Could you check a few things on this model? Use its own coordinates, in mm. Face numbers are marked on the shaded views. A direction names the side the tool comes from. Round coordinates to 2 decimals unless told otherwise and drop trailing zeros. Loops run counter-clockwise (first coordinate to the right, second up) from the corner with the lowest first, then second, coordinate; pieces in that order, holes last. Notation, with made-up numbers: (36, -14.5) -> (48, -14.5) arc R27 cw to (48, 9.5) -> close; hole circle Ø6 at (69, -24). An arc over 180 degrees is marked (long way). Write each question's results on one line, items separated by ' | '.
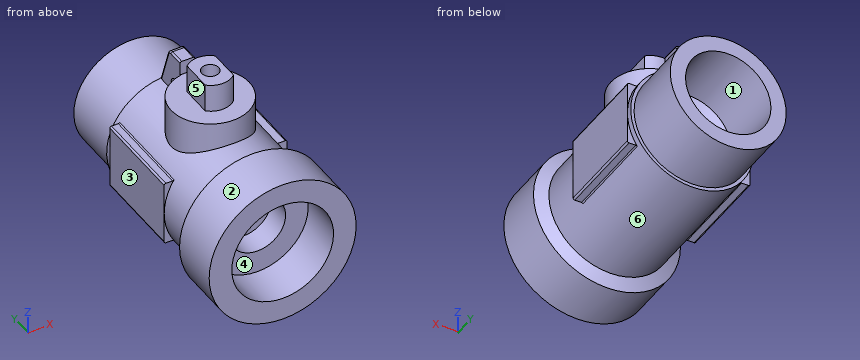
from build123d import *

# Parameters (mm, degrees)
SKETCH2_W                = 16.5
SKETCH2_H                = 11.5
BOSS_EXTRUDE1_DEPTH      = 2
BOSS_EXTRUDE2_DEPTH      = 4.5
BOSS_EXTRUDE2_DEPTH_BACK = 3
SKETCH3_R                = 6.925
BOSS_EXTRUDE6_DEPTH      = 1.3
BOSS_EXTRUDE6_DEPTH_BACK = 1.3
SKETCH4_R                = 1
FILLET2_R                = 0.3
FILLET4_R                = 0.3
FILLET7_R                = 0.3
FILLET8_R                = 0.3
FILLET9_R                = 0.3
FILLET10_R               = 0.3
FILLET11_R               = 0.3
FILLET12_R               = 0.3
SKETCH5_R                = 1.5
BOSS_EXTRUDE7_DEPTH      = 5
FILLET13_R               = 1


with BuildPart() as part:
    # Sketch1 → Revolve1 (revolve)
    with BuildSketch(Plane.XY, mode=Mode.PRIVATE) as revolve1_sk:
        Polygon((7.55, 45.85), (7.55, 33.85), (5, 32.85), (5, 28.85), (0, 28.85), (0, 12), (5, 12), (5, 7.7), (9, 7.7), (9, 0), (13, 0), (13, 9), (10.85, 10), (10.85, 34.85), (10.25, 34.85), (10.25, 45.85), align=None)
    revolve(revolve1_sk.sketch.rotate(Axis((0, 0, 0), (0, 1, 0)), 90), axis=Axis((0, 0, 0), (0, 1, 0)))

    # Sketch2 → Boss-Extrude1 (add)
    with BuildSketch(Plane.YZ.offset(10.85)):
        with Locations((25.6, 0)):
            Rectangle(SKETCH2_W, SKETCH2_H)
    boss_extrude1 = extrude(amount=-BOSS_EXTRUDE1_DEPTH)

    # Mirror1: Boss-Extrude1 across plane
    add(boss_extrude1.mirror(Plane(origin=(0, 0, 0), x_dir=(0, 0, 1), z_dir=(1, 0, 0))))

    # Sketch3 → Boss-Extrude2 (add, two sides: drawn at the far end of the back side and taken through both)
    with BuildSketch(Plane(origin=(0, 0, 10.85), x_dir=(0, -1, 0), z_dir=(0, 0, 1)).offset(-BOSS_EXTRUDE2_DEPTH_BACK)):
        with Locations(Location((-22, 0, 0), (0, 0, 90))):
            Circle(SKETCH3_R)
    extrude(amount=BOSS_EXTRUDE2_DEPTH + BOSS_EXTRUDE2_DEPTH_BACK)

    # Sketch4 → Boss-Extrude6 (add, two sides: drawn at the far end of the back side and taken through both)
    with BuildSketch(Plane(origin=(0, 0, 0), x_dir=(0, 0, -1), z_dir=(1, 0, 0)).offset(-BOSS_EXTRUDE6_DEPTH_BACK)):
        Polygon((-10.85, 34.85), (-17.85, 32.425), (-17.85, 28.925), (-15.35, 28.925), (-15.35, 27.925), (-10.25, 27.925), (-10.25, 34.85), align=None)
        with Locations((-12.35, 30.625)):
            Circle(SKETCH4_R, mode=Mode.SUBTRACT)
    extrude(amount=BOSS_EXTRUDE6_DEPTH + BOSS_EXTRUDE6_DEPTH_BACK)

    # Fillet2
    fillet2_edges = [part.edges().sort_by_distance(p)[0] for p in [
        (-9.201086892, 25.6, 5.75),
    ]]
    fillet(fillet2_edges, radius=FILLET2_R)

    # Fillet4
    fillet4_edges = [part.edges().sort_by_distance(p)[0] for p in [
        (10.85, 25.6, 5.75),
    ]]
    fillet(fillet4_edges, radius=FILLET4_R)

    # Fillet7
    fillet7_edges = [part.edges().sort_by_distance(p)[0] for p in [
        (10.85, 25.6, -5.75),
    ]]
    fillet(fillet7_edges, radius=FILLET7_R)

    # Fillet8
    fillet8_edges = [part.edges().sort_by_distance(p)[0] for p in [
        (-10.85, 25.6, -5.75),
    ]]
    fillet(fillet8_edges, radius=FILLET8_R)

    # Fillet9
    fillet9_edges = [part.edges().sort_by_distance(p)[0] for p in [
        (-10.85, 25.6, 5.75),
    ]]
    fillet(fillet9_edges, radius=FILLET9_R)

    # Fillet10
    # the kernel refuses this fillet: 0.3 mm, written as the material it takes off along each edge
    with BuildSketch(Plane(origin=(1.3, 33.175, 17.85), x_dir=(0, 0, -1), z_dir=(0, -1, 0))) as fillet10_piece_1:
        with BuildLine():
            CenterArc((FILLET10_R, -FILLET10_R), FILLET10_R, 90, 90)
            Line((0, -FILLET10_R), (0, 0))
            Line((0, 0), (FILLET10_R, 0))
        make_face()
    extrude(amount=5, mode=Mode.SUBTRACT)
    with BuildSketch(Plane(origin=(-1.3, 35.095506775, 10.141320648), x_dir=(0, -0.9449058020160995, -0.3273423671270065), z_dir=(0, -0.3273423671270065, 0.9449058020160995))) as fillet10_piece_2_section:
        with BuildLine():
            CenterArc((FILLET10_R, FILLET10_R), FILLET10_R, 180, 90)
            Line((0, FILLET10_R), (0, 0))
            Line((0, 0), (FILLET10_R, 0))
        make_face()
    fillet10_piece_2 = extrude(amount=8.908145854, mode=Mode.PRIVATE)
    fillet10_piece_2 = fillet10_piece_2 - Plane(origin=(0, 33.459049613, 0), x_dir=(0, 0, -1), z_dir=(0, 1, 0)) * Cylinder(10.85, 20, mode=Mode.PRIVATE)
    add(fillet10_piece_2, mode=Mode.SUBTRACT)
    with BuildSketch(Plane(origin=(-1.3, 33.175, 17.85), x_dir=(0, 0, -1), z_dir=(0, -1, 0))) as fillet10_piece_3:
        with BuildLine():
            CenterArc((FILLET10_R, FILLET10_R), FILLET10_R, 180, 90)
            Line((0, FILLET10_R), (0, 0))
            Line((0, 0), (FILLET10_R, 0))
        make_face()
    extrude(amount=5, mode=Mode.SUBTRACT)
    with BuildSketch(Plane(origin=(1.3, 35.095506775, 10.141320648), x_dir=(0, -0.9449058020160995, -0.3273423671270065), z_dir=(0, -0.3273423671270065, 0.9449058020160995))) as fillet10_piece_4_section:
        with BuildLine():
            CenterArc((FILLET10_R, -FILLET10_R), FILLET10_R, 90, 90)
            Line((0, -FILLET10_R), (0, 0))
            Line((0, 0), (FILLET10_R, 0))
        make_face()
    fillet10_piece_4 = extrude(amount=8.908145854, mode=Mode.PRIVATE)
    fillet10_piece_4 = fillet10_piece_4 - Plane(origin=(0, 33.459049613, 0), x_dir=(0, 0, -1), z_dir=(0, 1, 0)) * Cylinder(10.85, 20, mode=Mode.PRIVATE)
    add(fillet10_piece_4, mode=Mode.SUBTRACT)

    # Fillet11
    fillet11_edges = [part.edges().sort_by_distance(p)[0] for p in [
        (9.201086892, 25.6, -5.75),
    ]]
    fillet(fillet11_edges, radius=FILLET11_R)

    # Fillet12
    fillet12_edges = [part.edges().sort_by_distance(p)[0] for p in [
        (-9.201086892, 25.6, -5.75),
    ]]
    fillet(fillet12_edges, radius=FILLET12_R)

    # Sketch5 → Boss-Extrude7 (add)
    with BuildSketch(Plane.XY.offset(15.35)):
        with BuildLine():
            Line((-2.5, 19.25), (-2.5, 24.75))
            ThreePointArc((-2.5, 24.75), (0, 25.75), (2.5, 24.75))
            Line((2.5, 24.75), (2.5, 19.25))
            ThreePointArc((2.5, 19.25), (0, 18.25), (-2.5, 19.25))
        make_face()
        with Locations((0, 22)):
            Circle(SKETCH5_R, mode=Mode.SUBTRACT)
    extrude(amount=BOSS_EXTRUDE7_DEPTH)

    # Fillet13
    # the kernel refuses this fillet: 1 mm, written as the material it takes off along each edge
    with BuildSketch(Plane(origin=(-1.3, 31.713122021, 16.85), x_dir=(0, 0, 1), z_dir=(0, -1, 0))) as fillet13_piece_1:
        with BuildLine():
            CenterArc((0.7, -0.3), 0.3, 0, 90)
            Line((1, -0.3), (1, 0))
            Line((1, 0), (0.7, 0))
        make_face()
    revolve(axis=Axis((-1.3, 31.713122021, 16.85), (-1, 0, 0)), revolution_arc=70.892452859, mode=Mode.SUBTRACT)
    with BuildSketch(Plane(origin=(1.3, 31.713122021, 16.85), x_dir=(0, 0.9449058020160994, 0.32734236712700643), z_dir=(0, 0.32734236712700643, -0.9449058020160994))) as fillet13_piece_2:
        with BuildLine():
            CenterArc((0.7, -0.3), 0.3, 0, 90)
            Line((1, -0.3), (1, 0))
            Line((1, 0), (0.7, 0))
        make_face()
    revolve(axis=Axis((1.3, 31.713122021, 16.85), (1, 0, 0)), revolution_arc=70.892452859, mode=Mode.SUBTRACT)
    with BuildSketch(Plane(origin=(-1.3, 32.425, 17.85), x_dir=(0, 0.32734236712700615, -0.9449058020160995), z_dir=(1, 0, 0))) as fillet13_piece_3:
        with BuildLine():
            CenterArc((FILLET13_R * 0.711877979199, -FILLET13_R), FILLET13_R, 90, 70.892452859)
            Line((-FILLET13_R * 0.233027822817, -FILLET13_R * 0.672657632873), (0, 0))
            Line((0, 0), (FILLET13_R * 0.711877979199, 0))
        make_face()
    extrude(amount=2.6, mode=Mode.SUBTRACT)


solid = part.part
1) I want a section at B-B, the plane z = 12.35. Give the number of separate pieces and of enclosed holes in the cut face, plus the area to 3 significant figures.
Model answer:
separate pieces: 3 | enclosed holes: 0 | area: 234 mm2
2) If we mould it in two halves opening along Z, with no side actions, what happens to the marked faces 1, 2 and 3? For each: released by +Z, released by -Z, zero draft, split by the parting line, or undercut.
Model answer:
face 1: undercut | face 2: split by the parting line | face 3: zero draft
3) For the marked faces 4, 5 and 6, which set-ups out of +Z, -Z, +X, -X, +Y, -Y let a thin tool reach every point of the face, with its end or its side?
Model answer:
face 4: -Y | face 5: +Z, -X, +Y, -Y | face 6: none
4) I'm going to push flat-ended pins straight in: pin 1 (11 mm diameter, centred on x = 0, z = 0, fed in from +Y); pin 2 (1.5 mm diameter, centred on y = 22, z = 17.5, fed in from -X); pin 3 (0.6 mm diameter, centred on x = 10, y = 22, fed in from -Z). Where does each tip first touch, or does it pass through?
Model answer:
pin 1: stops at y = 33.05 | pin 2: stops at x = -2.5 | pin 3: stops at z = -5.75
5) I want a section at A-A, the plane y = 21. Write out the boundary of the cut face in (x, z).
Model answer:
outline: (-10.85, -5.45) arc R0.3 ccw to (-10.55, -5.75) -> (-9.37, -5.75) arc R0.3 cw to (-9.11, -5.89) arc R10.85 ccw to (9.11, -5.89) arc R0.3 cw to (9.37, -5.75) -> (10.55, -5.75) arc R0.3 ccw to (10.85, -5.45) -> (10.85, 5.45) arc R0.3 ccw to (10.55, 5.75) -> (9.2, 5.75) arc R10.85 ccw to (6.85, 8.41) -> (6.85, 15.35) -> (2.5, 15.35) -> (2.5, 20.35) -> (1.12, 20.35) -> (1.12, 15.35) -> (-1.12, 15.35) -> (-1.12, 20.35) -> (-2.5, 20.35) -> (-2.5, 15.35) -> (-6.85, 15.35) -> (-6.85, 8.41) arc R10.85 ccw to (-9.11, 5.89) arc R0.3 cw to (-9.37, 5.75) -> (-10.55, 5.75) arc R0.3 ccw to (-10.85, 5.45) -> close
6) I need wall thicknesses on line 1 (X direction, y = 3, z = 0); line 2 (Y direction, x = 0.55, z = 12.35) (3 decimals); line 3 (Y direction, x = -0.5, z = 16.5) (3 decimals). Which ranges of each line are inside material? Lowest first, please.
Model answer:
line 1: x = -13 to -9, 9 to 13 | line 2: y = 0 to 9.297, 15.097 to 29.625, 31.625 to 34.33 | line 3: y = 18.285 to 20.586, 23.414 to 25.715, 28.925 to 32.893
